```python
from build123d import *

# Parameters (mm, degrees)
SKETCH1_W           = 140
SKETCH1_H           = 30
BOSS_EXTRUDE1_DEPTH = 10
SKETCH2_R           = 5.5
CUT_EXTRUDE1_DEPTH  = 73.284161474


with BuildPart() as part:
    # Sketch1 → Boss-Extrude1 (new body)
    with BuildSketch(Plane(origin=(0, 0, 0), x_dir=(1, 0, 0), z_dir=(0, 1, 0))):
        Rectangle(SKETCH1_W, SKETCH1_H)
    extrude(amount=BOSS_EXTRUDE1_DEPTH)

    # Sketch2 → Cut-Extrude1 (cut, through all)
    with BuildSketch(Plane(origin=(0, 10, 0), x_dir=(1, 0, 0), z_dir=(0, 1, 0))):
        with Locations(Location((-60, 0, 0), (0, 0, 270))):
            Circle(SKETCH2_R)
        with Locations(Location((60, 0, 0), (0, 0, 270))):
            Circle(SKETCH2_R)
    extrude(amount=-CUT_EXTRUDE1_DEPTH, mode=Mode.SUBTRACT)

    # Sketch4 → M16 Tapped Hole1 (revolve, cut)
    with BuildSketch(Plane(origin=(0, 10, 0), x_dir=(0, 0, 1), z_dir=(1, 0, 0))):
        Polygon((0, 0), (0, 45), (7, 38), (7, 0), align=None)
    revolve(axis=Axis((0, 16.35, 0), (0, -1, 0)), mode=Mode.SUBTRACT)


solid = part.part
```
Could you check a few things on this model? Use its own coordinates, in mm. Coordinates: 2 decimals unless noted, no trailing zeros. Loops run counter-clockwise (first coordinate to the right, second up) from the corner with the lowest first, then second, coordinate; pieces in that order, holes last. Notation, with made-up numbers: M 86.5,80.5 L 140.5,80.5 A12 cw 140.5,89.5 Z; hole C 46,17.5 d5. An arc over 180 degrees is marked long. Put each result on its own line as item: value. Start each with the question number.
(1) Suppose I cut it at B-B on z = 0. Please give me the cut outline in (x, y).
(2) Thinking about a two-plate mould opening in Z: for faces 1 (the face through (2.681, 5.07, 6.466)), 2 (the face through (-1, 5, 15)), 3 (the face through (-1, 10, -10)), which applies, pulls with the +Z half, pulls with the -Z half, needs draft (parallel to the pull), parting line crosses it, or undercut?
(3) Suppose I cut it at C-C on y = 6. Please give me the cut outline in (x, z), then the cut area to 3 significant figures.
(4) I need wall thicknesses on line 1 (X direction, y = 4.25, z = 0); line 2 (Z direction, x = 0, y = 2.5); line 3 (X direction, y = 6.5, z = 1). Which ranges of each line are inside material? Lowest first, please. Write a range as from..to.
(5) Suppose I cut it at A-A on x = 0. Please give me the cut outline in (y, z), then the cut area to 3 significant figures.
(6) Suppose I cut it at D-D on x = -60. Please give me the cut outline in (y, z).
Solutions:
1. outline: M -70,0 L -65.5,0 L -65.5,10 L -70,10 Z; M -54.5,0 L -7,0 L -7,10 L -54.5,10 Z; M 7,0 L 54.5,0 L 54.5,10 L 7,10 Z; M 65.5,0 L 70,0 L 70,10 L 65.5,10 Z
2. face 1: undercut
2. face 2: pulls with the +Z half
2. face 3: needs draft
3. outline: M -70,-15 L 70,-15 L 70,15 L -70,15 Z; hole C -60,0 d11; hole C 0,0 d14; hole C 60,0 d11
3. area: 3,860 mm2
4. line 1: x = -70..-65.5, -54.5..-7, 7..54.5, 65.5..70
4. line 2: z = -15..-7, 7..15
4. line 3: x = -70..-65.41, -54.59..-6.93, 6.93..54.59, 65.41..70
5. outline: M 0,-15 L 10,-15 L 10,-7 L 0,-7 Z; M 0,7 L 10,7 L 10,15 L 0,15 Z
5. area: 160 mm2
6. outline: M 0,-15 L 10,-15 L 10,-5.5 L 0,-5.5 Z; M 0,5.5 L 10,5.5 L 10,15 L 0,15 Z
